Input: dimensioned drawing with shaded views. Units: mm. Origin: part minimum x, y, z. Round coordinates to 2 decimals unless told otherwise and drop trailing zeros. Write each loop counter-clockwise with the first axis right and the second up, starting at its lowest first coordinate (ties: lowest second). Pieces come first, ordered by that corner, then holes. Notation, with made-up numbers: (-30.75, 24.5) - (22.25, 24.5) arc R23 cw to (22.25, 49.5) - close; hole circle Ø7 at (-28.5, -18.75). An arc over 180 degrees is marked (long way). Write item = value, one per line. Start each with the question number.
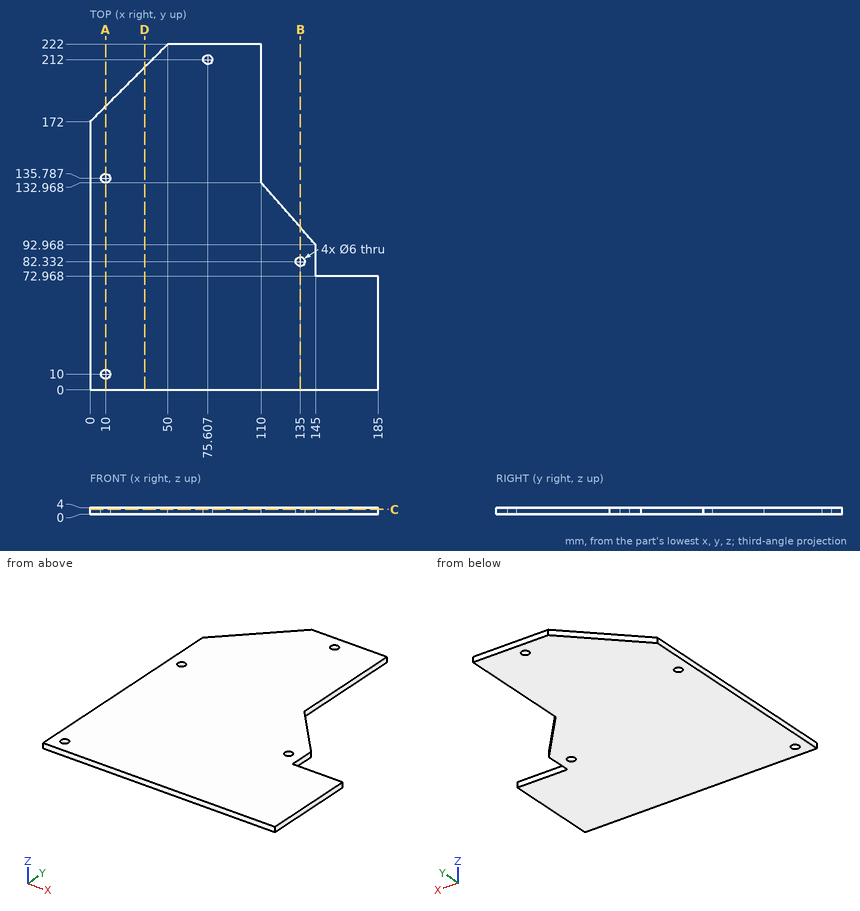
(1) Section A-A (x = 10). Return the cut outline in (y, z), plus the area to 3 significant figures.
(2) Section C-C (z = 3.05). Return the cut outline in (x, y).
(3) Section D-D (x = 35). Return the cut outline in (y, z).
(4) Contact query for flat-ended pins moving along their axis: P1, Ø2, axis at y = 186, z = 1.5, coming from the +X side; P2, Ø5, axis at x = 10, y = 10, coming from the +Z side. Output: stop coordinate, or through.
(5) Section B-B (x = 135). Return the cut outline in (y, z).
(6) Ray query, L1, parallel to Y at x = 169.5, z = 2.65; L2, parallel to X at y = 152, z = 3.1; L3, parallel to X at y = 212, z = 2.2 (1 decimal). Return the intervals inside material, ascending. Write a range as from..to.
Solution:
q1.outline = (0, 0) - (7, 0) - (7, 4) - (0, 4) - close; (13, 0) - (132.79, 0) - (132.79, 4) - (13, 4) - close; (138.79, 0) - (182, 0) - (182, 4) - (138.79, 4) - close
q1.area = 680 mm^2
q2.outline = (0, 0) - (185, 0) - (185, 72.97) - (145, 72.97) - (145, 92.97) - (110, 132.97) - (110, 222) - (50, 222) - (0, 172) - close; hole circle Ø6 at (10, 10); hole circle Ø6 at (10, 135.79); hole circle Ø6 at (75.61, 212); hole circle Ø6 at (135, 82.33)
q3.outline = (0, 0) - (207, 0) - (207, 4) - (0, 4) - close
q4.P1 = 110
q4.P2 = through
q5.outline = (0, 0) - (79.33, 0) - (79.33, 4) - (0, 4) - close; (85.33, 0) - (104.4, 0) - (104.4, 4) - (85.33, 4) - close
q6.L1 = 0..72.97
q6.L2 = 0..110
q6.L3 = 40..72.6, 78.6..110
